from build123d import *

# Parameters (mm, degrees)
ESQUISSE1_R               = 75
BOSS_EXTRU_1_DEPTH        = 22.2
CONG_1_R                  = 10
ESQUISSE2_W               = 14
ESQUISSE2_H               = 60
BOSS_EXTRU_2_DEPTH        = 28
ESQUISSE3_R               = 1
ENL_V_MAT_EXTRU_1_DEPTH   = 10
ESQUISSE5_W               = 12
ESQUISSE5_H               = 8
PASSAGE_CABLE_MG995_DEPTH = 118.34581373


with BuildPart() as part:
    # Esquisse1 → Boss.-Extru.1 (new body)
    with BuildSketch(Plane.XY):
        Circle(ESQUISSE1_R)
    extrude(amount=BOSS_EXTRU_1_DEPTH)

    # Congé1
    cong_1_edges = [part.edges().sort_by_distance(p)[0] for p in [
        (-75, 0, 22.2),
    ]]
    fillet(cong_1_edges, radius=CONG_1_R)

    # Esquisse2 → Boss.-Extru.2 (add)
    with BuildSketch(Plane.XY.offset(22.2)):
        with Locations((-27.5, 0)):
            Rectangle(ESQUISSE2_W, ESQUISSE2_H)
        with Locations((27.5, 0)):
            Rectangle(ESQUISSE2_W, ESQUISSE2_H)
    extrude(amount=BOSS_EXTRU_2_DEPTH)

    # Esquisse3 → Enlèv. mat.-Extru.1 (cut)
    with BuildSketch(Plane.XY.offset(50.2)):
        with Locations((-24.2, 5.65)):
            Circle(ESQUISSE3_R)
        with Locations(Location((-24.2, -5.65, 0), (0, 0, 180))):
            Circle(ESQUISSE3_R)
        with Locations((24.2, -5.65)):
            Circle(ESQUISSE3_R)
        with Locations(Location((24.2, 5.65, 0), (0, 0, 180))):
            Circle(ESQUISSE3_R)
    extrude(amount=-ENL_V_MAT_EXTRU_1_DEPTH, mode=Mode.SUBTRACT)

    # Esquisse5 → Passage cable MG995 (cut, through all)
    with BuildSketch(Plane(origin=(0, 0, 0), x_dir=(0, 0, -1), z_dir=(1, 0, 0))):
        with Locations((-28.2, 0)):
            Rectangle(ESQUISSE5_W, ESQUISSE5_H)
    extrude(amount=PASSAGE_CABLE_MG995_DEPTH, mode=Mode.SUBTRACT)


solid = part.part
For this review, take the finished solid that the model builds, in its own axes (mm). A direction names the side the tool comes from. Round coordinates to 2 decimals unless told otherwise and drop trailing zeros. Write each loop counter-clockwise with the first axis right and the second up, starting at its lowest first coordinate (ties: lowest second). Pieces come first, ordered by that corner, then holes. Notation, with made-up numbers: M -4,43 L 41,43 A8 ccw 41,50 Z; hole C -14.75,60.5 d10. An arc over 180 degrees is marked long. Write item = value, one per line. Start each with the question number.
(1) Clearance check with flat-ended pins moving along their axes: pin 1 Ø11 at (x, z) = (-29, 40.5) entering from +Y; pin 2 Ø1 at (x, y) = (-24, 6) entering from +Z; pin 3 Ø8 at (y, z) = (-13, 38) entering from +X. State where each tip first meets the part, or that it passes through.
(2) For line 1 along Y through (x, z) = (-24.2, 42.75); line 2 along X through (y, z) = (5, 47); line 3 along X through (y, z) = (10.5, 42.5), list the stretches that pass through material, from the lowest coordinate up.
(3) We need section A-A (y = 0). Give the boundary of the cut face in (x, z).
(4) We need section B-B (x = 0). Give the boundary of the cut face in (y, z).
(5) The part is to be moulded in two halves that separate along Z. For faces 1 (the face through (27, 0, 34.2)), 2 (the face through (-28, 0, 50.2)), 3 (the face through (27, 30, 36)), 4 (the face through (27, 4, 28)), say which applies: +Z half, -Z half, draft (parallel to the pull), parting line (faces both ways), or undercut.
(6) For faces 5 (the face through (27, -30, 36)), 6 (the face through (-34.5, 0, 36)), 7 (the face through (-28, 30, 36)), 8 (the face through (27, -4, 28)), 9 (the face through (34.5, 0, 36)), list the 3-axis set-ups (+Z, -Z, +X, -X, +Y, -Y) from which the entire face can be reached by the end or side of a thin tool; tool diameter is ignored.
(7) We need section D-D (z = 17.5). Give the boundary of the cut face in (x, y).
(8) We need section C-C (z = 6). Give the boundary of the cut face in (x, y), then the cut area to 3 significant figures.
Results found:
q1.pin_1 = 30
q1.pin_2 = 40.2
q1.pin_3 = 34.5
q2.line_1 = -30 to -6.65, -4.65 to 4.65, 6.65 to 30
q2.line_2 = -34.5 to -24.96, -23.44 to -20.5, 20.5 to 23.44, 24.96 to 34.5
q2.line_3 = -34.5 to -20.5, 20.5 to 34.5
q3.outline = M -75,0 L 75,0 L 75,12.2 A10 ccw 65,22.2 L -20.5,22.2 L -20.5,50.2 L -34.5,50.2 L -34.5,22.2 L -65,22.2 A10 ccw -75,12.2 Z; M 20.5,34.2 L 34.5,34.2 L 34.5,50.2 L 20.5,50.2 Z
q4.outline = M -75,0 L 75,0 L 75,12.2 A10 ccw 65,22.2 L -65,22.2 A10 ccw -75,12.2 Z
q5.face_1 = undercut
q5.face_2 = +Z half
q5.face_3 = draft
q5.face_4 = undercut
q6.face_5 = +Z, +X, -X, -Y
q6.face_6 = +Z, -X, +Y, -Y
q6.face_7 = +Z, +X, -X, +Y
q6.face_8 = +X
q6.face_9 = +Z, +X, +Y, -Y
q7.outline = C 0,0 d146.96
q8.outline = C 0,0 d150
q8.area = 17,700 mm²
